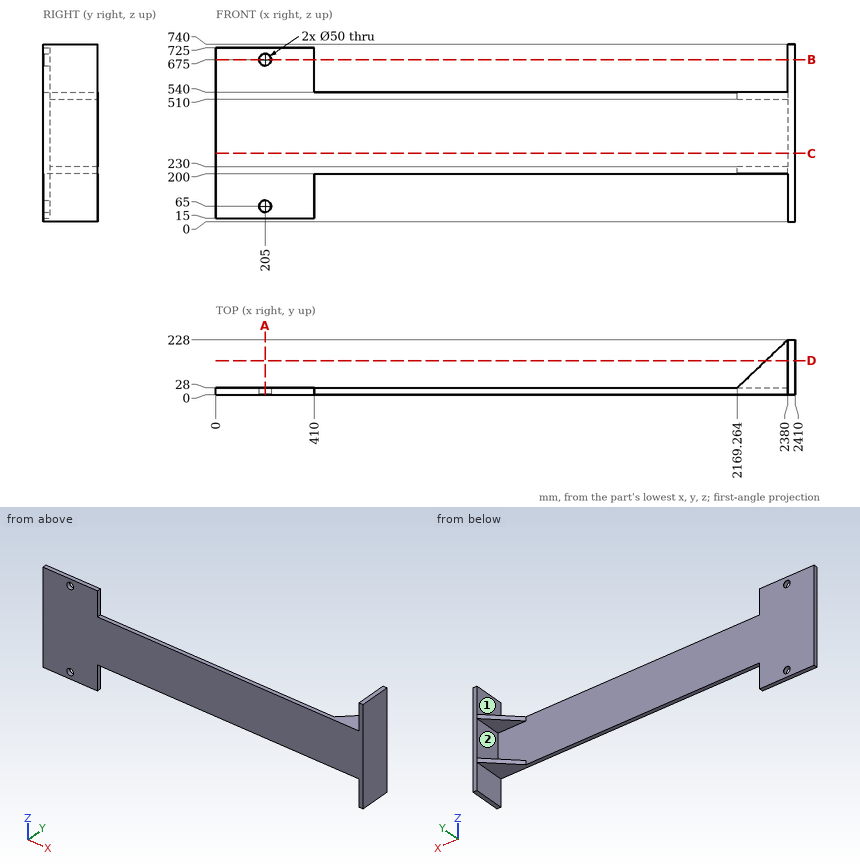
Geometry check sheet. Reference: drawing and pictorial views, mm from the part's lowest x, y, z. Round coordinates to 2 decimals unless told otherwise and drop trailing zeros. Loops run counter-clockwise (first coordinate to the right, second up) from the corner with the lowest first, then second, coordinate; pieces in that order, holes last. Notation, with made-up numbers: (60.5, -12.75) - (118.5, -12.75) arc R25 cw to (118.5, 2.25) - close; hole circle Ø3 at (69.25, 22). An arc over 180 degrees is marked (long way). Use a Markdown table: item, result. Add a question column.
1. Section check D-D, the plane y = 142. Record the boundary of the cut face in (x, z).
2. Gauge pin test, flat ends, axial feed: pin 1 (14 mm diameter, centred on x = 246.5, y = 8.5, fed in from +Z); pin 2 (22.5 mm diameter, centred on x = 271, y = 13.5, fed in from -Z); pin 3 (1 mm diameter, centred on x = 1902, z = 345.5, fed in from +Y). Record the tip position at first contact, or that the pin passes through.
3. Section check C-C, the plane z = 284.5. Record the boundary of the cut face in (x, y), plus the area to 3 significant figures.
4. Section check B-B, the plane z = 675. Record the boundary of the cut face in (x, y).
5. Thickness scan on probe 1 along X at (y, z) = (9, 65); probe 2 along Z at (x, y) = (205, 10); probe 3 along X at (y, z) = (71, 691). Record the ranges inside material, lowest first. Write a range as [from, to].
6. Release check for a two-part mould opening along Z. For the marked faces 1 and 2 record: released by +Z, released by -Z, zero draft, split by the parting line, or undercut.
7. Section check A-A, the plane x = 205. Record the boundary of the cut face in (y, z).
Checks:
| question | item | result |
|---|---|---|
| 1 | outline | (2289.38, 200) - (2380, 200) - (2380, 0) - (2410, 0) - (2410, 740) - (2380, 740) - (2380, 540) - (2289.38, 540) - (2289.38, 510) - (2380, 510) - (2380, 230) - (2289.38, 230) - close |
| 2 | pin 1 | stops at z = 725 |
| 2 | pin 2 | stops at z = 15 |
| 2 | pin 3 | stops at y = 28 |
| 3 | outline | (0, 0) - (2410, 0) - (2410, 228) - (2380, 228) - (2380, 28) - (0, 28) - close |
| 3 | area | 73,500 mm^2 |
| 4 | outline | (0, 0) - (180, 0) - (180, 28) - (0, 28) - close; (230, 0) - (410, 0) - (410, 28) - (230, 28) - close; (2380, 0) - (2410, 0) - (2410, 228) - (2380, 228) - close |
| 5 | probe 1 | x = [0, 180], [230, 410], [2380, 2410] |
| 5 | probe 2 | z = [15, 40], [90, 650], [700, 725] |
| 5 | probe 3 | x = [2380, 2410] |
| 6 | face 1 | zero draft |
| 6 | face 2 | undercut |
| 7 | outline | (0, 15) - (28, 15) - (28, 40) - (0, 40) - close; (0, 90) - (28, 90) - (28, 650) - (0, 650) - close; (0, 700) - (28, 700) - (28, 725) - (0, 725) - close |
